```python
from build123d import *

# Parameters (mm, degrees)
SKETCH1_3_W         = 9.525
SKETCH1_3_H         = 3.175
BOSS_EXTRUDE2_DEPTH = 19.250000108
SKETCH3_R           = 2.286
CUT_EXTRUDE1_DEPTH  = 41.930807193
FILLET1_R           = 1.8


with BuildPart() as part:
    # Sketch1_3 → Boss-Extrude2 (new, symmetric)
    with BuildSketch(Plane.XY):
        Polygon((17.662500108, -17.662500108), (-17.662500108, -17.662500108), (-17.662500108, -1.27), (-20.837500108, -1.27), (-20.837500108, -4.445), (-20.837500108, -20.837500108), (20.837500108, -20.837500108), (20.837500108, -4.445), (20.837500108, -1.27), (17.662500108, -1.27), align=None)
        with Locations((-25.600000108, -2.8575)):
            Rectangle(SKETCH1_3_W, SKETCH1_3_H)
        with Locations((25.600000108, -2.8575)):
            Rectangle(SKETCH1_3_W, SKETCH1_3_H)
    extrude(amount=BOSS_EXTRUDE2_DEPTH, both=True)

    # Sketch3 → Cut-Extrude1 (cut, through all)
    with BuildSketch(Plane(origin=(0, -1.27, 0), x_dir=(1, 0, 0), z_dir=(0, 1, 0))):
        with Locations(Location((-25.600000108, 12.7, 0), (0, 0, 270))):
            Circle(SKETCH3_R)
        with Locations(Location((-25.600000108, -12.7, 0), (0, 0, 270))):
            Circle(SKETCH3_R)
        with Locations(Location((25.600000108, 12.7, 0), (0, 0, 270))):
            Circle(SKETCH3_R)
        with Locations(Location((25.600000108, -12.7, 0), (0, 0, 270))):
            Circle(SKETCH3_R)
    extrude(amount=-CUT_EXTRUDE1_DEPTH, mode=Mode.SUBTRACT)

    # Fillet1
    fillet1_edges = [part.edges().sort_by_distance(p)[0] for p in [
        (-17.662500108, -17.662500108, 0),
        (17.662500108, -17.662500108, 0),
        (20.837500108, -4.445, 0),
        (-20.837500108, -4.445, 0),
    ]]
    fillet(fillet1_edges, radius=FILLET1_R)


solid = part.part
```
Can you work these out from the model? Positions are in its coordinate system, mm. A direction names the side the tool comes from. Coordinates: 2 decimals unless noted, no trailing zeros. Loops run counter-clockwise (first coordinate to the right, second up) from the corner with the lowest first, then second, coordinate; pieces in that order, holes last. Notation, with made-up numbers: (-5.75, -3) -> (34.25, -3) arc R22 cw to (34.25, 34) -> close; hole circle Ø6 at (61.5, -28). An arc over 180 degrees is marked (long way). Answer as a JSON object with one key per item and string values.
1) If I drill on line 1 (X direction, y = -3.05, z = 12.7); line 2 (Z direction, x = -25.6, y = -2.05); line 3 (X direction, y = -14.25, z = 14), over which ranges is the centre line in solid material (lowest first)?
Results:
{"line 1": "x = -30.36 to -27.89, -23.31 to -17.66, 17.66 to 23.31, 27.89 to 30.36", "line 2": "z = -19.25 to -14.99, -10.41 to 10.41, 14.99 to 19.25", "line 3": "x = -20.84 to -17.66, 17.66 to 20.84"}
2) Thinking about a two-plate mould opening in X: for faces 4 (the face through (2, -18, -19.25)), 5 (the face through (-20.838, -13, 0)), 6 (the face through (-27.63, -2.84, 13.75)), which applies, pulls with the +X half, pulls with the -X half, needs draft (parallel to the pull), parting line crosses it, or undercut?
Results:
{"face 4": "needs draft", "face 5": "pulls with the -X half", "face 6": "undercut"}
3) Imagine slicing it at D-D (y = -7). Please give me the cut outline in (x, z), then the cut area to 3 significant figures.
Results:
{"outline": "(-20.84, -19.25) -> (-17.66, -19.25) -> (-17.66, 19.25) -> (-20.84, 19.25) -> close; (17.66, -19.25) -> (20.84, -19.25) -> (20.84, 19.25) -> (17.66, 19.25) -> close", "area": "244 mm^2"}
4) For P1, Ø4.5, axis at y = -7, z = -6, coming from the -X side (3 decimals); P2, Ø2, axis at y = -8.5, z = 10.5, coming from the -X side; P3, Ø7.5, axis at y = -13.5, z = 4, coming from the +X side, each with a flat end and sliding along its axis, tell me the tip position at first contact or that it passes through.
Results:
{"P1": "stops at x = -21.635", "P2": "stops at x = -20.84", "P3": "stops at x = 20.84"}
5) Imagine slicing it at B-B (z = 12.7). Please give me the cut outline in (x, y) (1 decimal), then the cut area to 3 significant figures.
Results:
{"outline": "(-30.4, -4.4) -> (-27.9, -4.4) -> (-27.9, -1.3) -> (-30.4, -1.3) -> close; (-23.3, -4.4) -> (-22.6, -4.4) arc R1.8 cw to (-20.8, -6.2) -> (-20.8, -20.8) -> (20.8, -20.8) -> (20.8, -6.2) arc R1.8 cw to (22.6, -4.4) -> (23.3, -4.4) -> (23.3, -1.3) -> (17.7, -1.3) -> (17.7, -15.9) arc R1.8 cw to (15.9, -17.7) -> (-15.9, -17.7) arc R1.8 cw to (-17.7, -15.9) -> (-17.7, -1.3) -> (-23.3, -1.3) -> close; (27.9, -4.4) -> (30.4, -4.4) -> (30.4, -1.3) -> (27.9, -1.3) -> close", "area": "271 mm^2"}
6) For faces 1 (the face through (0, -20.838, 0)), 2 (the face through (0, -17.663, 0)), 3 (the face through (26, -4.445, 0)), which set-ups out of +Z, -Z, +X, -X, +Y, -Y let a thin tool reach every point of the face, with its end or its side?
Results:
{"face 1": "+Z, -Z, +X, -X, -Y", "face 2": "+Z, -Z, +Y", "face 3": "+Z, -Z, +X, -Y"}
7) Imagine slicing it at A-A (y = -2.75). Please give me the cut outline in (x, z).
Results:
{"outline": "(-30.36, -19.25) -> (-17.66, -19.25) -> (-17.66, 19.25) -> (-30.36, 19.25) -> close; (17.66, -19.25) -> (30.36, -19.25) -> (30.36, 19.25) -> (17.66, 19.25) -> close; hole circle Ø4.57 at (-25.6, -12.7); hole circle Ø4.57 at (-25.6, 12.7); hole circle Ø4.57 at (25.6, -12.7); hole circle Ø4.57 at (25.6, 12.7)"}
8) Imagine slicing it at C-C (x = -25.6). Please give me the cut outline in (y, z) (3 decimals).
Results:
{"outline": "(-4.445, -19.25) -> (-1.27, -19.25) -> (-1.27, -14.986) -> (-4.445, -14.986) -> close; (-4.445, -10.414) -> (-1.27, -10.414) -> (-1.27, 10.414) -> (-4.445, 10.414) -> close; (-4.445, 14.986) -> (-1.27, 14.986) -> (-1.27, 19.25) -> (-4.445, 19.25) -> close"}
